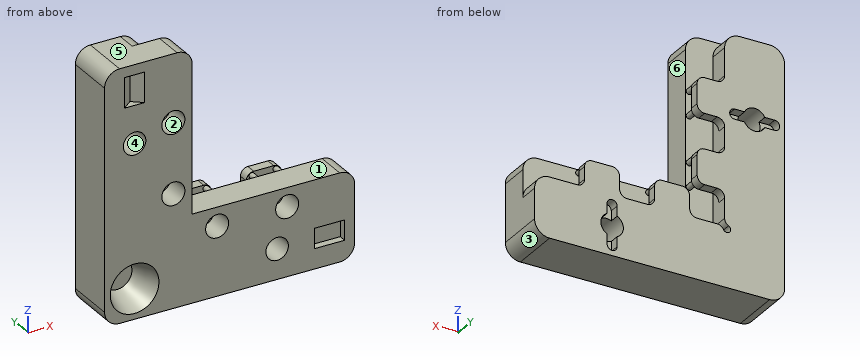
from build123d import *

# Parameters (mm, degrees)
PAD006_DEPTH     = 4
PAD002_DEPTH     = 10
SKETCH005_R      = 2.25
POCKET001_DEPTH  = 10.001
BOX_W            = 50
BOX_H            = 50
BOX_DEPTH        = 2
HOLE_D           = 3.4
HOLE_DEPTH       = 6
HOLE_CBORE_D     = 4.6
HOLE_CBORE_DEPTH = 5
HOLE_TIPS_R      = 1.7
SKETCH017_R      = 0.55
PAD009_DEPTH     = 4
POCKET007_DEPTH  = 2
POCKET008_DEPTH  = 6
SKETCH022_W      = 1.5
SKETCH022_H      = 4
POCKET009_DEPTH  = 6
FILLET_R         = 3


with BuildPart() as setscrewbackplatecutbody:
    # Sketch013 → Pad006 (new body, symmetric)
    with BuildSketch(Plane.XZ.offset(-11.5)):
        with BuildLine():
            Line((19, 13.5), (19, 16))
            ThreePointArc((20.5, 17.5), (19.43934, 17.06066), (19, 16))
            Line((20.5, 17.5), (24.5, 17.5))
            ThreePointArc((26, 16), (25.56066, 17.06066), (24.5, 17.5))
            Line((26, 16), (26, 13.5))
            ThreePointArc((26, 13.5), (26.43934, 12.43934), (27.5, 12))
            Line((27.5, 12), (31.5, 12))
            ThreePointArc((31.5, 12), (32.56066, 12.43934), (33, 13.5))
            Line((33, 13.5), (33, 16))
            ThreePointArc((34.5, 17.5), (33.43934, 17.06066), (33, 16))
            Line((34.5, 17.5), (38.5, 17.5))
            ThreePointArc((40, 16), (39.56066, 17.06066), (38.5, 17.5))
            Line((40, 16), (40, 13.5))
            ThreePointArc((40, 13.5), (40.43934, 12.43934), (41.5, 12))
            Line((41.5, 12), (70, 12))
            Line((70, 12), (70, 23.387521))
            Line((70, 23.387521), (23.387521, 70))
            Line((23.387521, 70), (12, 70))
            Line((12, 70), (12, 41.5))
            ThreePointArc((12, 41.5), (12.43934, 40.43934), (13.5, 40))
            Line((13.5, 40), (16, 40))
            ThreePointArc((17.5, 38.5), (17.06066, 39.56066), (16, 40))
            Line((17.5, 38.5), (17.5, 34.5))
            ThreePointArc((16, 33), (17.06066, 33.43934), (17.5, 34.5))
            Line((16, 33), (13.5, 33))
            ThreePointArc((13.5, 33), (12.43934, 32.56066), (12, 31.5))
            Line((12, 31.5), (12, 27.5))
            ThreePointArc((12, 27.5), (12.43934, 26.43934), (13.5, 26))
            Line((13.5, 26), (16, 26))
            ThreePointArc((17.5, 24.5), (17.06066, 25.56066), (16, 26))
            Line((17.5, 24.5), (17.5, 20.5))
            ThreePointArc((16, 19), (17.06066, 19.43934), (17.5, 20.5))
            Line((16, 19), (13.5, 19))
            ThreePointArc((13.5, 19), (12.43934, 18.56066), (12, 17.5))
            Line((12, 17.5), (12, 13.5))
            ThreePointArc((11.221376, 12.229989), (11.789849, 12.755154), (12, 13.5))
            ThreePointArc((11.221376, 12.229989), (11.031264, 11.031264), (12.229989, 11.221376))
            ThreePointArc((13.5, 12), (12.755154, 11.789849), (12.229989, 11.221376))
            Line((13.5, 12), (17.5, 12))
            ThreePointArc((17.5, 12), (18.56066, 12.43934), (19, 13.5))
        make_face()
    extrude(amount=PAD006_DEPTH, both=True)


with BuildPart() as obj1:
    # Sketch003 (on DatumPlane) → Pad002 (new body)
    with BuildSketch(Plane.XZ.offset(-1.5)):
        with BuildLine():
            Line((3, 0), (47, 0))
            ThreePointArc((47, 0), (49.12132, 0.87868), (50, 3))
            Line((50, 3), (50, 14.5))
            ThreePointArc((50, 14.5), (49.12132, 16.62132), (47, 17.5))
            Line((47, 17.5), (17.5, 17.5))
            Line((17.5, 17.5), (17.5, 47))
            ThreePointArc((17.5, 47), (16.62132, 49.12132), (14.5, 50))
            Line((14.5, 50), (3, 50))
            ThreePointArc((3, 50), (0.87868, 49.12132), (0, 47))
            Line((0, 47), (0, 3))
            ThreePointArc((0, 3), (0.87868, 0.87868), (3, 0))
        make_face()
    extrude(amount=-PAD002_DEPTH)

    # Sketch005 (on DatumPlane) → Pocket001 (cut, through all)
    with BuildSketch(Plane.XZ.offset(-1.5)):
        with Locations((34.5, 6)):
            Circle(SKETCH005_R)
        with Locations((6, 34.5)):
            Circle(SKETCH005_R)
    extrude(amount=-POCKET001_DEPTH, mode=Mode.SUBTRACT)

    # Box → Box (cut)
    with BuildSketch(Plane(origin=(12, 9.5, 12), x_dir=(1, 0, 0), z_dir=(0, -1, 0))):
        with Locations((25, 25)):
            Rectangle(BOX_W, BOX_H)
    extrude(amount=BOX_DEPTH, mode=Mode.SUBTRACT)

    # Boolean003: cut SetscrewBackplateCutBody
    add(setscrewbackplatecutbody.part, mode=Mode.SUBTRACT)

    # Hole
    with Locations(Plane.XZ.offset(-1.5)):
        with Locations((36.5, 13.75), (22.5, 13.75), (13.75, 22.5), (13.75, 36.5)):
            CounterBoreHole(HOLE_D / 2, HOLE_CBORE_D / 2, HOLE_CBORE_DEPTH, depth=HOLE_DEPTH)

    # Hole tips → Hole tip 1 section 0
    with BuildSketch(Plane.XZ.offset(-7.5), mode=Mode.PRIVATE) as hole_tip_1_s0:
        with Locations((36.5, 13.75)):
            Circle(HOLE_TIPS_R)
    loft([hole_tip_1_s0.sketch, Vertex(36.5, 8.521463, 13.75)], mode=Mode.SUBTRACT)

    # Hole tips → Hole tip 2 section 0
    with BuildSketch(Plane.XZ.offset(-7.5), mode=Mode.PRIVATE) as hole_tip_2_s0:
        with Locations((22.5, 13.75)):
            Circle(HOLE_TIPS_R)
    loft([hole_tip_2_s0.sketch, Vertex(22.5, 8.521463, 13.75)], mode=Mode.SUBTRACT)

    # Hole tips → Hole tip 3 section 0
    with BuildSketch(Plane.XZ.offset(-7.5), mode=Mode.PRIVATE) as hole_tip_3_s0:
        with Locations((13.75, 22.5)):
            Circle(HOLE_TIPS_R)
    loft([hole_tip_3_s0.sketch, Vertex(13.75, 8.521463, 22.5)], mode=Mode.SUBTRACT)

    # Hole tips → Hole tip 4 section 0
    with BuildSketch(Plane.XZ.offset(-7.5), mode=Mode.PRIVATE) as hole_tip_4_s0:
        with Locations((13.75, 36.5)):
            Circle(HOLE_TIPS_R)
    loft([hole_tip_4_s0.sketch, Vertex(13.75, 8.521463, 36.5)], mode=Mode.SUBTRACT)

    # Sketch017 (on DatumPlane) → Pad009 (join)
    with BuildSketch(Plane.XZ.offset(-11.5)):
        with Locations((38.9, 16.8)):
            Circle(SKETCH017_R)
        with Locations((34.1, 16.8)):
            Circle(SKETCH017_R)
        with Locations((24.9, 16.8)):
            Circle(SKETCH017_R)
        with Locations((20.1, 16.8)):
            Circle(SKETCH017_R)
        with Locations((16.8, 20.1)):
            Circle(SKETCH017_R)
        with Locations((16.8, 24.9)):
            Circle(SKETCH017_R)
        with Locations((16.8, 34.1)):
            Circle(SKETCH017_R)
        with Locations((16.8, 38.9)):
            Circle(SKETCH017_R)
    extrude(amount=PAD009_DEPTH)

    # Sketch019 (on DatumPlane) → Pocket007 (cut)
    with BuildSketch(Plane.XZ.offset(-11.5)):
        with BuildLine():
            ThreePointArc((35.5, 10), (34.5, 11), (33.5, 10))
            Line((33.5, 10), (33.5, 2))
            ThreePointArc((33.5, 2), (34.5, 1), (35.5, 2))
            Line((35.5, 2), (35.5, 10))
        make_face()
        with BuildLine():
            ThreePointArc((10, 33.5), (11, 34.5), (10, 35.5))
            Line((10, 35.5), (2, 35.5))
            ThreePointArc((2, 35.5), (1, 34.5), (2, 33.5))
            Line((2, 33.5), (10, 33.5))
        make_face()
    extrude(amount=POCKET007_DEPTH, mode=Mode.SUBTRACT)

    # Sketch021 → Pocket008 (cut)
    with BuildSketch(Plane.XY.offset(48)):
        Polygon((4, 1.5), (8, 1.5), (6, 3.1), align=None)
    extrude(amount=-POCKET008_DEPTH, mode=Mode.SUBTRACT)

    # Sketch022 → Pocket009 (cut)
    with BuildSketch(Plane.YZ.offset(48)):
        with Locations((2.25, 6)):
            Rectangle(SKETCH022_W, SKETCH022_H)
    extrude(amount=-POCKET009_DEPTH, mode=Mode.SUBTRACT)

    # Cone001 → Cone001 (revolve, cut)
    with BuildSketch(Plane(origin=(6, 1.5, 6), x_dir=(-1, 0, 0), z_dir=(0, 0, -1))):
        Polygon((0, 0), (4.869, 0), (2.983, 6), (0, 6), align=None)
    revolve(axis=Axis((6, 1.5, 6), (0, 1, 0)), mode=Mode.SUBTRACT)

    # Fillet
    fillet_edges = [obj1.edges().sort_by_distance(p)[0] for p in [
        (12, 9.5, 50),
        (50, 9.5, 12),
    ]]
    fillet(fillet_edges, radius=FILLET_R)


solid = obj1.part
Read the model definition and answer for the solid it produces. Units are mm, in the model's axes. Face numbers are marked on the shaded views. A direction names the side the tool comes from. Give positions to 0.01 mm unless a question says otherwise; leave off trailing zeros. Write each loop counter-clockwise with the first axis right and the second up, starting at its lowest first coordinate (ties: lowest second). Pieces come first, ordered by that corner, then holes. Notation, with made-up numbers: (-4.75, 81) - (37.25, 81) arc R38 ccw to (37.25, 120) - close; hole circle Ø8 at (-22.75, 10.25). An arc over 180 degrees is marked (long way). Answer in a Markdown table with one row per item. Add a question column.
Item 1: Section B-B, the plane z = 46 is taken. Write down the section's boundary in (x, y).
Item 2: Find the intervals of material crossed by L1, parallel to Z at x = 13.75, y = 5.3; L2, parallel to Z at x = 22.5, y = 3.75; L3, parallel to X at y = 5, z = 23 (3 decimals), in increasing order.
Item 3: Flat-ended cylindrical pins translate along their axes: P1, Ø1.4, axis at x = 23, z = 13.5, coming from the -Y side; P2, Ø0.6, axis at y = 11, z = 36, coming from the +X side; P3, Ø2, axis at x = 15, y = 10, coming from the +Z side. Find the tip coordinate at first contact, or state that the pin passes through.
Item 4: Section A-A, the plane z = 22.5 is taken. Write down the section's boundary in (x, y).
Item 5: A tool of negligible diameter and unlimited length cuts with its end or side. For the marked faces 1, 2 and 3, from which of +Z, -Z, +X, -X, +Y, -Y can it reach the whole face along a straight path? Write none if from no direction.
Item 6: Section C-C, the plane y = 5.5 is taken. Write down the section's boundary in (x, z), and give its area (3 significant figures).
Item 7: Determine the mould class of the marked faces 4, 5 and 6 for opening direction X: pulls with the +X half, pulls with the -X half, needs draft (parallel to the pull), parting line crosses it, or undercut.
Item 8: Section D-D, the plane x = 23 is taken. Write down the section's boundary in (y, z) (3 decimals), and give its area (3 significant figures).
Recorded:
| question | item | result |
|---|---|---|
| 1 | outline | (0, 1.5) - (4, 1.5) - (6, 3.1) - (8, 1.5) - (17.5, 1.5) - (17.5, 7.5) - (12, 7.5) - (12, 11.5) - (0, 11.5) - close |
| 2 | L1 | z = 0 to 20.2, 24.8 to 34.2, 38.8 to 50 |
| 2 | L2 | z = 0 to 11.45, 16.05 to 17.5 |
| 2 | L3 | x = 0 to 11.505, 15.995 to 17.5 |
| 3 | P1 | stops at y = 9.5 |
| 3 | P2 | stops at x = 17.5 |
| 3 | P3 | stops at z = 40 |
| 4 | outline | (0, 1.5) - (11.45, 1.5) - (11.45, 6.5) - (12.05, 6.5) - (12.05, 7.5) - (12, 7.5) - (12, 9.5) - (17.5, 9.5) - (17.5, 11.5) - (0, 11.5) - close; (15.45, 6.5) - (16.05, 6.5) - (16.05, 1.5) - (17.5, 1.5) - (17.5, 7.5) - (15.45, 7.5) - close |
| 5 | face 1 | +Z, +X, +Y, -Y |
| 5 | face 2 | -Y |
| 5 | face 3 | -Z, +X, +Y, -Y |
| 6 | outline | (0, 3) arc R3 ccw to (3, 0) - (47, 0) arc R3 ccw to (50, 3) - (50, 14.5) arc R3 ccw to (47, 17.5) - (17.5, 17.5) - (17.5, 47) arc R3 ccw to (14.5, 50) - (3, 50) arc R3 ccw to (0, 47) - close; hole circle Ø7.22 at (6, 6); hole circle Ø4.5 at (6, 34.5); hole circle Ø4.6 at (13.75, 22.5); hole circle Ø4.6 at (13.75, 36.5); hole circle Ø4.6 at (22.5, 13.75); hole circle Ø4.5 at (34.5, 6); hole circle Ø4.6 at (36.5, 13.75) |
| 6 | area | 1,290 mm2 |
| 7 | face 4 | undercut |
| 7 | face 5 | needs draft |
| 7 | face 6 | pulls with the +X half |
| 8 | outline | (1.5, 0) - (11.5, 0) - (11.5, 17.5) - (9.5, 17.5) - (9.5, 12) - (7.5, 12) - (7.5, 12.125) - (6.5, 12.125) - (6.5, 11.505) - (1.5, 11.505) - close; (1.5, 15.995) - (6.5, 15.995) - (6.5, 15.375) - (7.5, 15.375) - (7.5, 17.5) - (1.5, 17.5) - close |
| 8 | area | 138 mm2 |
